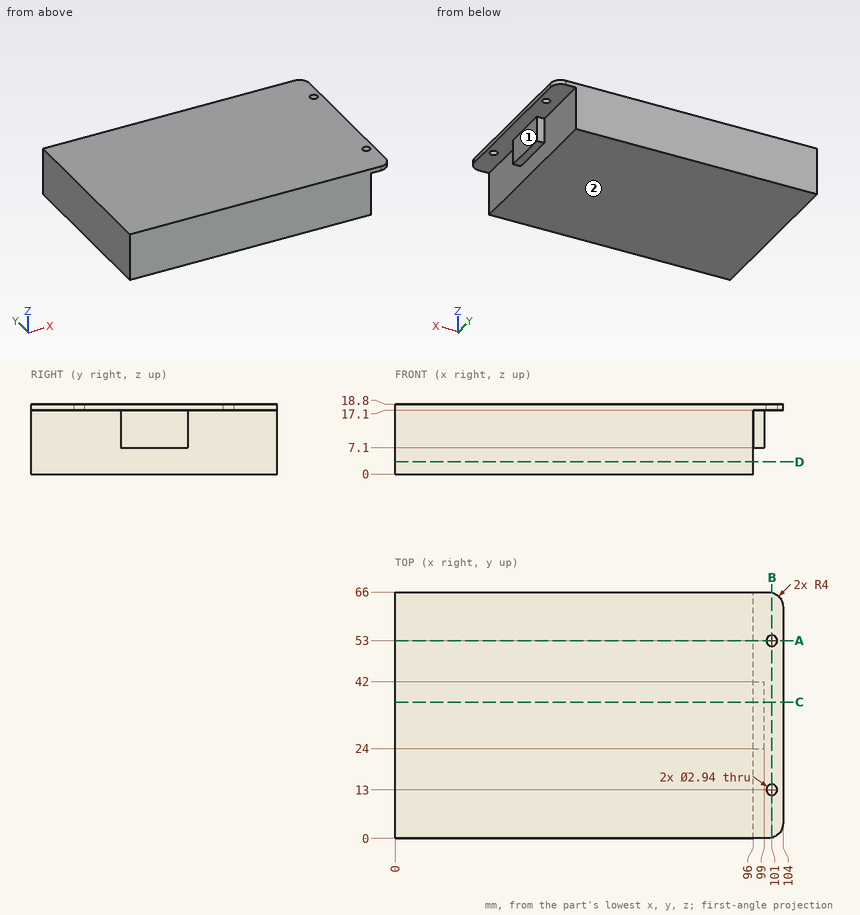
The figure shows three views and two pictorial views of one solid part (mm, origin at its lowest corner). Answer the questions. A direction names the side the tool comes from. Coordinates: 2 decimals unless noted, no trailing zeros. Order: outer loops, then holes, each group sorted by start corner. A loop starts at its lowest first (then second) coordinate and runs counter-clockwise, first axis right, second up.
Q1. A cutting plane is placed at B-B, the plane x = 101. Write down the section's boundary in (y, z), and give its area (3 significant figures).
Q2. Consider line 1 (Y direction, x = 101, z = 17.8); line 2 (X direction, y = 17, z = 4); line 3 (X direction, y = 41, z = 10). Determine where each line is inside the solid, lowest interval first.
Q3. Which of the six approach directions +Z, -Z, +X, -X, +Y, -Y give full straight-line access (tool end or side, diameter ignored) to the marked faces 1 and 2?
Q4. Given P1, Ø0.9, axis at x = 97.5, z = 11, coming from the -Y side; P2, Ø2.5, axis at x = 101.5, y = 33.5, coming from the -Z side; P3, Ø5, axis at y = 24, z = 6.5, coming from the -X side; P4, Ø3.5, axis at x = 98, y = 35.5, coming from the -Z side, each flat-ended and moving along its own axis, determine where each tip first touches the part or whether it passes through.
Q5. A cutting plane is placed at C-C, the plane y = 36.5. Write down the section's boundary in (x, z), and give its area (3 significant figures).
Q6. A cutting plane is placed at D-D, the plane z = 3.25. Write down the section's boundary in (x, y).
Q7. A cutting plane is placed at A-A, the plane y = 53. Write down the section's boundary in (x, z), and give its area (3 significant figures).
Answers follow:
1. outline: (0.13, 17.1) - (11.53, 17.1) - (11.53, 18.8) - (0.13, 18.8) - close; (14.47, 17.1) - (51.53, 17.1) - (51.53, 18.8) - (14.47, 18.8) - close; (54.47, 17.1) - (65.87, 17.1) - (65.87, 18.8) - (54.47, 18.8) - close
1. area: 102 mm2
2. line 1: y = 0.13 to 11.53, 14.47 to 51.53, 54.47 to 65.87
2. line 2: x = 0 to 96
2. line 3: x = 0 to 99
3. face 1: -Z, +X, +Y, -Y
3. face 2: -Z, +X, -X, +Y, -Y
4. P1: stops at y = 24
4. P2: stops at z = 17.1
4. P3: stops at x = 0
4. P4: stops at z = 7.1
5. outline: (0, 0) - (96, 0) - (96, 7.1) - (99, 7.1) - (99, 17.1) - (104, 17.1) - (104, 18.8) - (0, 18.8) - close
5. area: 1,850 mm2
6. outline: (0, 0) - (96, 0) - (96, 66) - (0, 66) - close
7. outline: (0, 0) - (96, 0) - (96, 17.1) - (99.53, 17.1) - (99.53, 18.8) - (0, 18.8) - close; (102.47, 17.1) - (104, 17.1) - (104, 18.8) - (102.47, 18.8) - close
7. area: 1,810 mm2
